from build123d import *

# Parameters (mm, degrees)
SKETCH2_W           = 44
SKETCH2_H           = 40.022099447
SKETCH2_W_2         = 36
SKETCH2_H_2         = 32.022099447
EXTRUDE_THIN1_DEPTH = 950
SKETCH3_R           = 3.35
CUT_EXTRUDE1_DEPTH  = 41.022099448


with BuildPart() as part:
    # Sketch2 → Extrude-Thin1 (new body, symmetric)
    with BuildSketch(Plane.XY):
        with Locations((0.028084851, 0.02246788)):
            Rectangle(SKETCH2_W, SKETCH2_H)
        with Locations((0.028084851, 0.02246788)):
            Rectangle(SKETCH2_W_2, SKETCH2_H_2, mode=Mode.SUBTRACT)
    extrude(amount=EXTRUDE_THIN1_DEPTH, both=True)

    # Sketch3 → Cut-Extrude1 (cut, through all)
    with BuildSketch(Plane(origin=(0, 20.033517604, 0), x_dir=(1, 0, 0), z_dir=(0, 1, 0))):
        with Locations((0, 815.652483779)):
            Circle(SKETCH3_R)
        with Locations((0, 765.652483779)):
            Circle(SKETCH3_R)
        with Locations((0, 715.652483779)):
            Circle(SKETCH3_R)
        with Locations((0, 665.652483779)):
            Circle(SKETCH3_R)
        with Locations((0, 615.652483779)):
            Circle(SKETCH3_R)
        with Locations((0, 565.652483779)):
            Circle(SKETCH3_R)
        with Locations((0, 515.652483779)):
            Circle(SKETCH3_R)
        with Locations((0, 465.652483779)):
            Circle(SKETCH3_R)
        with Locations((0, 415.652483779)):
            Circle(SKETCH3_R)
        with Locations((0, 365.652483779)):
            Circle(SKETCH3_R)
        with Locations((0, 315.652483779)):
            Circle(SKETCH3_R)
        with Locations((0, 265.652483779)):
            Circle(SKETCH3_R)
        with Locations((0, 215.652483779)):
            Circle(SKETCH3_R)
        with Locations((0, 165.652483779)):
            Circle(SKETCH3_R)
        with Locations((0, 115.652483779)):
            Circle(SKETCH3_R)
        with Locations((0, 65.652483779)):
            Circle(SKETCH3_R)
        with Locations((0, 15.652483779)):
            Circle(SKETCH3_R)
        with Locations((0, -34.347516221)):
            Circle(SKETCH3_R)
        with Locations((0, -84.347516221)):
            Circle(SKETCH3_R)
        with Locations((0, -134.347516221)):
            Circle(SKETCH3_R)
        with Locations((0, -184.347516221)):
            Circle(SKETCH3_R)
        with Locations((0, -234.347516221)):
            Circle(SKETCH3_R)
        with Locations((0, -284.347516221)):
            Circle(SKETCH3_R)
        with Locations((0, -334.347516221)):
            Circle(SKETCH3_R)
        with Locations((0, -384.347516221)):
            Circle(SKETCH3_R)
        with Locations((0, -434.347516221)):
            Circle(SKETCH3_R)
        with Locations((0, -484.347516221)):
            Circle(SKETCH3_R)
        with Locations((0, -534.347516221)):
            Circle(SKETCH3_R)
        with Locations((0, -584.347516221)):
            Circle(SKETCH3_R)
        with Locations((0, -634.347516221)):
            Circle(SKETCH3_R)
        with Locations((0, -684.347516221)):
            Circle(SKETCH3_R)
        with Locations((0, -734.347516221)):
            Circle(SKETCH3_R)
        with Locations((0, -784.347516221)):
            Circle(SKETCH3_R)
        with Locations((0, -834.347516221)):
            Circle(SKETCH3_R)
    extrude(amount=-CUT_EXTRUDE1_DEPTH, mode=Mode.SUBTRACT)


solid = part.part
Here's how the part is built. I have some questions about the finished solid (model axes, mm). A direction names the side the tool comes from. Coordinates: 2 decimals unless noted, no trailing zeros. Order: outer loops, then holes, each group sorted by start corner. A loop starts at its lowest first (then second) coordinate and runs counter-clockwise, first axis right, second up. Notation, with made-up numbers: (11.25, -30.5) - (25.25, -30.5) arc R19 cw to (25.25, -24.5) - close; hole circle Ø5 at (36.5, 17). An arc over 180 degrees is marked (long way). Use CSV: the item, a comma, the result in double quotes. Start each with the question number.
1. Please list where these lines run through material, in increasing order: line 1 (Y direction, x = -1, z = 45); line 2 (X direction, y = 0.5, z = -285). Write a range as from..to.
2. If we mould it in two halves opening along Y, with no side actions, what happens to faces 1 (the face through (0, 20.034, 13)), 2 (the face through (18.028, 0, 13)), 3 (the face through (0, -17, 950))? For each: +Y half, -Y half, draft (parallel to the pull), parting line (faces both ways), or undercut.
3. For faces 4 (the face through (0, -17, -950)), 5 (the face through (0, -15.989, 13)), which set-ups out of +Z, -Z, +X, -X, +Y, -Y let a thin tool reach every point of the face, with its end or its side?
4. I'm going to push a flat-ended pin straight in: pin 1 (5.5 mm diameter, centred on x = 0, z = -265.65, fed in from +Y). Where does the tip first touch, or does it pass through?
5. Suppose I cut it at A-A on y = -7. List the corners of the cut face in (x, z) for me.
Output:
1,line 1,"y = -19.99..-15.99, 16.03..20.03"
1,line 2,"x = -21.97..-17.97, 18.03..22.03"
2,face 1,"+Y half"
2,face 2,"undercut"
2,face 3,"draft"
3,face 4,"-Z, +X, -X, +Y, -Y"
3,face 5,"+Z, -Z"
4,pin 1,"passes through"
5,outline,"(-21.97, -950) - (-17.97, -950) - (-17.97, 950) - (-21.97, 950) - close; (18.03, -950) - (22.03, -950) - (22.03, 950) - (18.03, 950) - close"
